Build history of the part. All positions in model axes, mm. Face numbers are marked on the shaded views. A direction names the side the tool comes from. Round coordinates to 2 decimals unless told otherwise and drop trailing zeros. Order: outer loops, then holes, each group sorted by start corner. A loop starts at its lowest first (then second) coordinate and runs counter-clockwise, first axis right, second up. Notation, with made-up numbers: M -15.5,-1 L 35.5,-1 A18 ccw 35.5,31 Z; hole C 81,79 d3. An arc over 180 degrees is marked long. One line per question, with ' | ' between items. Start each with the question number.
from build123d import *

# Parameters (mm, degrees)
F1_DEPTH = 5
F2_DEPTH = 15
F3_DEPTH = 35
F4_R     = 3
F4_R_2   = 1.5
F5_DEPTH = 2
F4_R_3   = 4
F6_DEPTH = 0.25
F7_DEPTH = 25


# Not quite as in the source:
# - a feature names something its author has since deleted; it is built from what else it names


with BuildPart() as f1:
    # F0 (on Front) → F1 (new body)
    with BuildSketch(Plane.XZ):
        with BuildLine():
            Line((7, 2), (7, 10))
            ThreePointArc((7, 10), (0, 17), (-7, 10))
            Line((-7, 10), (-7, 2))
            Line((-7, 2), (7, 2))
        make_face()
        with BuildLine():
            ThreePointArc((3.3166247904, 15), (0, 4), (-3.3166247904, 15))
            Line((-3.3166247904, 15), (3.3166247904, 15))
        make_face(mode=Mode.SUBTRACT)
    extrude(amount=-F1_DEPTH)

    # F0 (on Front) → F2 (join)
    with BuildSketch(Plane.XZ):
        Polygon((15, 2), (7, 2), (-7, 2), (-15, 2), (-15, 0), (15, 0), align=None)
    extrude(amount=-F2_DEPTH)

    # F0 (on Front) → F3 (join)
    with BuildSketch(Plane.XZ):
        Polygon((15, 2), (7, 2), (-7, 2), (-15, 2), (-15, 0), (15, 0), align=None)
    extrude(amount=F3_DEPTH)

    # F4 (on face) → F5 (join)
    with BuildSketch(Plane.XY.offset(2)):
        with Locations((12, -18.75)):
            Circle(F4_R)
        with Locations((12, -18.75)):
            Circle(F4_R_2, mode=Mode.SUBTRACT)
    extrude(amount=F5_DEPTH)

    # F4 (on face) → F6 (join)
    with BuildSketch(Plane.XY.offset(2)):
        with Locations((0, -30)):
            Circle(F4_R_3)
        with Locations((0, -30)):
            Circle(F4_R_2, mode=Mode.SUBTRACT)
    extrude(amount=F6_DEPTH)

    # F4 (on face) → F7 (cut)
    with BuildSketch(Plane.XY.offset(2)):
        with Locations((-12, -21.25)):
            Circle(F4_R_2)
        with Locations((0, -30)):
            Circle(F4_R_2)
        with Locations((12, -18.75)):
            Circle(F4_R_2)
    extrude(amount=-F7_DEPTH, mode=Mode.SUBTRACT)


solid = f1.part
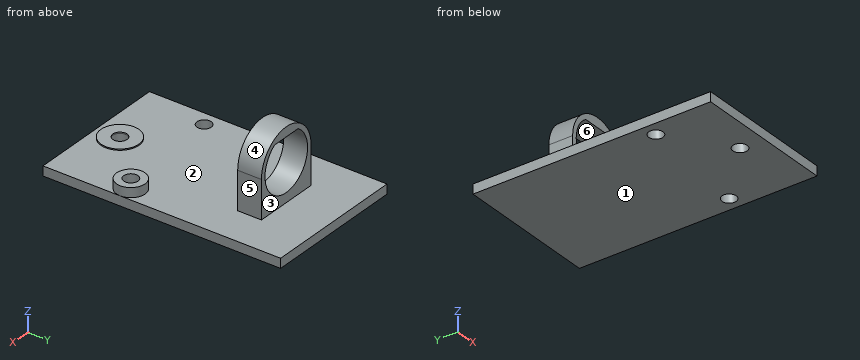
Item 1: Wall check: line 1 along Y through (x, z) = (0, 1.35); line 2 along Z through (x, y) = (0, 2.85); line 3 along Y through (x, z) = (12, 3.65). Give the ranges that are in metal, low to high. Write a range as [from, to].
Item 2: Cut at D-D on x = -12. Write the cut outline in (y, z).
Item 3: Cut at B-B on x = -1. Write the cut outline in (y, z), then the cut area to 3 significant figures.
Item 4: Tool access for the marked faces 4, 5 and 6: list every direction of +Z, -Z, +X, -X, +Y, -Y with a clear straight run to the whole face (end or side of a thin tool).
Item 5: Flat gauge pins, fed straight in: pin 1 (5 mm diameter, centred on x = 7.5, z = 15, fed in from +Y); pin 2 (1 mm diameter, centred on x = 3, y = -25, fed in from +Z); pin 3 (10 mm diameter, centred on x = 1.5, y = -28.5, fed in from +Z). Where does each tip first touch, or does it go through?
Item 6: Cut at A-A on x = 12. Write the cut outline in (y, z).
Item 7: Cut at C-C on z = 9.25. Write the cut outline in (x, y).
Item 8: Two-plate mould, pull along Y, no slides. Class the marked faces 1, 2 and 3: +Y half, -Y half, draft (parallel to the pull), parting line (faces both ways), or undercut.
Results found:
1) line 1: y = [-35, -31.5], [-28.5, 15] | line 2: z = [0, 4], [15, 17] | line 3: y = [-21.75, -20.25], [-17.25, -15.75]
2) outline: M -35,0 L -22.75,0 L -22.75,2 L -35,2 Z; M -19.75,0 L 15,0 L 15,2 L -19.75,2 Z
3) outline: M -35,0 L -31.12,0 L -31.12,2.25 L -33.87,2.25 L -33.87,2 L -35,2 Z; M -28.88,0 L 15,0 L 15,2 L 5,2 L 5,4.08 L 0,4.08 L 0,2 L -26.13,2 L -26.13,2.25 L -28.88,2.25 Z; M 0,15 L 5,15 L 5,16.93 L 0,16.93 Z | area: 117 mm^2
4) face 4: +Z, +Y, -Y | face 5: +Z, +X, +Y, -Y | face 6: +Y, -Y
5) pin 1: stops at y = 5 | pin 2: stops at z = 2 | pin 3: stops at z = 2.25
6) outline: M -35,0 L -20.25,0 L -20.25,4 L -21.75,4 L -21.75,2 L -35,2 Z; M -17.25,0 L 15,0 L 15,2 L -15.75,2 L -15.75,4 L -17.25,4 Z
7) outline: M -7,0 L -5.95,0 L -5.95,5 L -7,5 Z; M 5.95,0 L 7,0 L 7,5 L 5.95,5 Z
8) face 1: draft | face 2: undercut | face 3: +Y half
